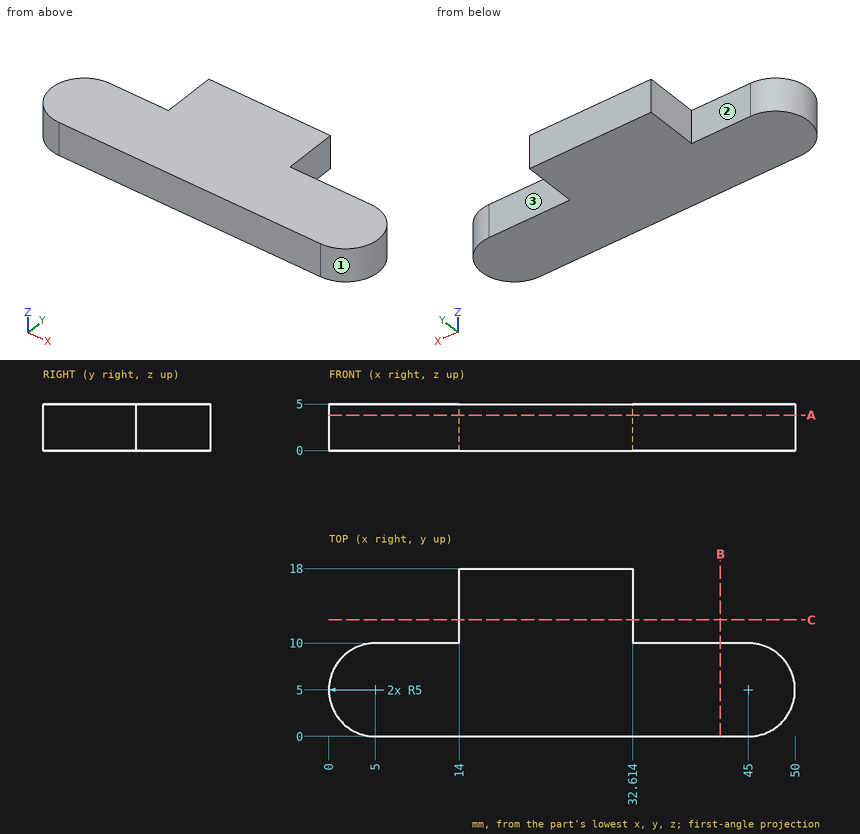
Print and shaded views of the part. All mm, measured from the part's lowest x, y and z. A direction names the side the tool comes from. Round coordinates to 2 decimals unless told otherwise and drop trailing zeros. Write each loop counter-clockwise with the first axis right and the second up, starting at its lowest first coordinate (ties: lowest second). Pieces come first, ordered by that corner, then holes. Notation, with made-up numbers: (-23.75, -1.5) - (14.25, -1.5) arc R27 ccw to (14.25, 22.5) - close; hole circle Ø11 at (36.25, 22). An arc over 180 degrees is marked (long way). Write each question's results on one line, items separated by ' | '. Start each with the question number.
Item 1: Drop flat-ended pins along their axis: P1, Ø2, axis at y = 2, z = 3.5, coming from the -X side; P2, Ø1.5, axis at y = 9.5, z = 3.5, coming from the -X side; P3, Ø1.5, axis at y = 14, z = 2.5, coming from the +X side. Give the stop position or say it passes through.
Item 2: Which spindle directions (+Z, -Z, +X, -X, +Y, -Y) get a long thin tool onto all of the face, cutting with end or side? Do the marked faces 1, 2 and 3. Say none if no direction does.
Item 3: Saw through at C-C (y = 12.5). Write the cut outline in (x, z).
Item 4: Saw through at B-B (x = 42). Write the cut outline in (y, z).
Item 5: Wall check: L1, parallel to Y at x = 12, z = 4.5; L2, parallel to X at y = 14.75, z = 0.9; L3, parallel to X at y = 8.5, z = 4.5. Give the ranges that are in metal, low to high. Write a range as [from, to].
Item 6: Saw through at A-A (z = 3.8). Write the cut outline in (x, y).
Results are:
1) P1: stops at x = 0.42 | P2: stops at x = 1.69 | P3: stops at x = 32.61
2) face 1: +Z, -Z, +X | face 2: +Z, -Z, -X, +Y | face 3: +Z, -Z, +X, +Y
3) outline: (14, 0) - (32.61, 0) - (32.61, 5) - (14, 5) - close
4) outline: (0, 0) - (10, 0) - (10, 5) - (0, 5) - close
5) L1: y = [0, 10] | L2: x = [14, 32.61] | L3: x = [1.43, 48.57]
6) outline: (5, 0) - (45, 0) arc R5 ccw to (45, 10) - (32.61, 10) - (32.61, 18) - (14, 18) - (14, 10) - (5, 10) arc R5 ccw to start
